Part model, mm, in its own coordinate system. A direction names the side the tool comes from. Give positions to 0.01 mm unless a question says otherwise; leave off trailing zeros. Order: outer loops, then holes, each group sorted by start corner. A loop starts at its lowest first (then second) coordinate and runs counter-clockwise, first axis right, second up. Notation, with made-up numbers: (58, 54) - (101, 54) arc R21 ccw to (101, 72) - close; hole circle Ø11 at (80.5, 18.25). An arc over 180 degrees is marked (long way). Use a Markdown table: item, result. Add a question column.
from build123d import *

# Parameters (mm, degrees)
SKETCH1_W           = 23.83
SKETCH1_H           = 1
BOSS_EXTRUDE1_DEPTH = 21.5
SKETCH2_R           = 1.325
BOSS_EXTRUDE2_DEPTH = 14.25
BOSS_EXTRUDE4_DEPTH = 8
SKETCH5_W           = 21.949336604
SKETCH5_H           = 2.5
BOSS_EXTRUDE5_DEPTH = 50
SKETCH6_R           = 4.25
SKETCH6_R_2         = 1.05
CUT_EXTRUDE1_DEPTH  = 83.099025573
FILLET1_R           = 7
FILLET2_R           = 7
FILLET3_R           = 7
BOSS_EXTRUDE6_START = 41
BOSS_EXTRUDE6_DEPTH = 41


with BuildPart() as part:
    # Sketch1 → Boss-Extrude1 (new body)
    with BuildSketch(Plane(origin=(0, 0, 0), x_dir=(1, 0, 0), z_dir=(0, 1, 0))):
        Rectangle(SKETCH1_W, SKETCH1_H)
    extrude(amount=BOSS_EXTRUDE1_DEPTH)

    # Sketch2 → Boss-Extrude2 (add, symmetric)
    with BuildSketch(Plane(origin=(0, 10.75, 0), x_dir=(1, 0, 0), z_dir=(0, 1, 0))):
        with Locations(Location((-11.915, 0, 0), (0, 0, 270))):
            Circle(SKETCH2_R)
        with Locations(Location((11.915, 0, 0), (0, 0, 270))):
            Circle(SKETCH2_R)
    extrude(amount=BOSS_EXTRUDE2_DEPTH, both=True)

    # Sketch4 → Boss-Extrude4 (add, symmetric)
    with BuildSketch(Plane(origin=(0, 0, 0), x_dir=(0, 0, -1), z_dir=(1, 0, 0))):
        Polygon((-0.5, 17.927447783), (-0.5, 21.5), (-12.5, 33.75), (-35.5, 33.75), (-35.5, 31.25), (-13.550663396, 31.25), align=None)
        Polygon((-0.5, 0), (-0.5, 3.572552217), (-13.550663396, -9.75), (-35.5, -9.75), (-35.5, -12.25), (-12.5, -12.25), align=None)
    extrude(amount=BOSS_EXTRUDE4_DEPTH, both=True)

    # Sketch5 → Boss-Extrude5 (add)
    with BuildSketch(Plane.ZY.offset(8)):
        with Locations((24.525331698, 32.5)):
            Rectangle(SKETCH5_W, SKETCH5_H)
        with Locations((24.525331698, -11)):
            Rectangle(SKETCH5_W, SKETCH5_H)
    extrude(amount=BOSS_EXTRUDE5_DEPTH)

    # Sketch6 → Cut-Extrude1 (cut, through all)
    with BuildSketch(Plane(origin=(0, 33.75, 0), x_dir=(1, 0, 0), z_dir=(0, 1, 0))):
        with Locations(Location((-47.025331698, -24.525331698, 0), (0, 0, 270))):
            Circle(SKETCH6_R)
        with Locations(Location((-54.025331698, -24.525331698, 0), (0, 0, 270))):
            Circle(SKETCH6_R_2)
        with Locations(Location((-47.025331698, -17.525331698, 0), (0, 0, 270))):
            Circle(SKETCH6_R_2)
        with Locations(Location((-40.025331698, -24.525331698, 0), (0, 0, 270))):
            Circle(SKETCH6_R_2)
        with Locations(Location((-47.025331698, -31.525331698, 0), (0, 0, 270))):
            Circle(SKETCH6_R_2)
        with BuildLine():
            ThreePointArc((-58, -24.525331743), (-54.785594092, -16.765069336), (-47.025331698, -13.550663396))
            Line((-47.025331698, -13.550663396), (-58, -13.550663396))
            Line((-58, -13.550663396), (-58, -24.525331743))
        make_face()
        with BuildLine():
            ThreePointArc((-47.025331698, -35.5), (-54.78559406, -32.285594092), (-58, -24.525331743))
            Line((-58, -24.525331743), (-58, -35.5))
            Line((-58, -35.5), (-47.025331698, -35.5))
        make_face()
    extrude(amount=-CUT_EXTRUDE1_DEPTH, mode=Mode.SUBTRACT)

    # Fillet1
    # the kernel refuses this fillet: 7 mm, written as the material it adds along each edge
    with BuildSketch(Plane(origin=(-8, -12.25, 13.550663396), x_dir=(-1, 0, 0), z_dir=(0, 1, 0))) as fillet1_piece_1_section:
        with BuildLine():
            CenterArc((FILLET1_R, -FILLET1_R), FILLET1_R, 90, 90)
            Line((0, -FILLET1_R), (0, 0))
            Line((0, 0), (FILLET1_R, 0))
        make_face()
    fillet1_piece_1 = extrude(amount=2.5, mode=Mode.PRIVATE)
    fillet1_piece_1 = split(fillet1_piece_1, bisect_by=Plane(origin=(-10.015975833, -11.661011889, 11.923032054), z_dir=(0, 0.699779834816443, 0.7143585813751185)), keep=Keep.TOP, mode=Mode.PRIVATE)
    fillet1_piece_1 = split(fillet1_piece_1, bisect_by=Plane(origin=(-10.015975833, -9.911562302, 13.708928508), z_dir=(0, -0.699779834816443, -0.7143585813751185)), keep=Keep.TOP, mode=Mode.PRIVATE)
    add(fillet1_piece_1)
    with BuildSketch(Plane(origin=(-8, -12.25, 13.550663396), x_dir=(-1, 0, 0), z_dir=(0, 1, 0))) as fillet1_piece_2_section:
        with BuildLine():
            CenterArc((FILLET1_R, -FILLET1_R), FILLET1_R, 90, 90)
            Line((0, -FILLET1_R), (0, 0))
            Line((0, 0), (FILLET1_R, 0))
        make_face()
    fillet1_piece_2 = extrude(amount=20, mode=Mode.PRIVATE)
    fillet1_piece_2 = split(fillet1_piece_2, bisect_by=Plane(origin=(-8.812454151, -9.294822672, 9.605132414), z_dir=(0, 0.699779834816443, 0.7143585813751185)), keep=Keep.TOP, mode=Mode.PRIVATE)
    fillet1_piece_2 = split(fillet1_piece_2, bisect_by=Plane(origin=(-8.812454151, -9.75, 10.768831879), z_dir=(0, 1, 0)), keep=Keep.TOP, mode=Mode.PRIVATE)
    fillet1_piece_2 = split(fillet1_piece_2, bisect_by=Plane(origin=(-8.812454151, -7.545373085, 11.391028867), z_dir=(0, -0.699779834816443, -0.7143585813751185)), keep=Keep.TOP, mode=Mode.PRIVATE)
    add(fillet1_piece_2)
    with BuildSketch(Plane(origin=(-8, 33.75, 13.550663396), x_dir=(0, 0, -1), z_dir=(0, -1, 0))) as fillet1_piece_3_section:
        with BuildLine():
            CenterArc((FILLET1_R, -FILLET1_R), FILLET1_R, 90, 90)
            Line((0, -FILLET1_R), (0, 0))
            Line((0, 0), (FILLET1_R, 0))
        make_face()
    fillet1_piece_3 = extrude(amount=2.5, mode=Mode.PRIVATE)
    fillet1_piece_3 = split(fillet1_piece_3, bisect_by=Plane(origin=(-10.015975833, 31.411562301, 13.708928507), z_dir=(0, 0.6997798348164432, -0.7143585813751182)), keep=Keep.TOP, mode=Mode.PRIVATE)
    fillet1_piece_3 = split(fillet1_piece_3, bisect_by=Plane(origin=(-10.015975833, 33.161011889, 11.923032054), z_dir=(0, -0.699779834816443, 0.7143585813751185)), keep=Keep.TOP, mode=Mode.PRIVATE)
    add(fillet1_piece_3)
    with BuildSketch(Plane(origin=(-8, 33.75, 13.550663396), x_dir=(0, 0, -1), z_dir=(0, -1, 0))) as fillet1_piece_4_section:
        with BuildLine():
            CenterArc((FILLET1_R, -FILLET1_R), FILLET1_R, 90, 90)
            Line((0, -FILLET1_R), (0, 0))
            Line((0, 0), (FILLET1_R, 0))
        make_face()
    fillet1_piece_4 = extrude(amount=20, mode=Mode.PRIVATE)
    fillet1_piece_4 = split(fillet1_piece_4, bisect_by=Plane(origin=(-8.812454159, 29.045373088, 11.39102887), z_dir=(0, 0.6997798348164432, -0.7143585813751182)), keep=Keep.TOP, mode=Mode.PRIVATE)
    fillet1_piece_4 = split(fillet1_piece_4, bisect_by=Plane(origin=(-8.812454159, 30.794822675, 9.605132416), z_dir=(0, -0.699779834816443, 0.7143585813751185)), keep=Keep.TOP, mode=Mode.PRIVATE)
    fillet1_piece_4 = split(fillet1_piece_4, bisect_by=Plane(origin=(-8.812454159, 31.25, 10.768831882), z_dir=(0, -1, 0)), keep=Keep.TOP, mode=Mode.PRIVATE)
    add(fillet1_piece_4)
    # the kernel refuses this fillet: 7 mm, written as the material it takes off along each edge
    with BuildSketch(Plane(origin=(8, 7.75, 35.5), x_dir=(0, 0, -1), z_dir=(0, -1, 0))) as fillet1_2_piece_1:
        with BuildLine():
            CenterArc((FILLET1_R, -FILLET1_R), FILLET1_R, 90, 90)
            Line((0, -FILLET1_R), (0, 0))
            Line((0, 0), (FILLET1_R, 0))
        make_face()
    extrude(amount=37.5, mode=Mode.SUBTRACT)
    with BuildSketch(Plane(origin=(8, 51.25, 35.5), x_dir=(-1, 0, 0), z_dir=(0, -1, 0))) as fillet1_2_piece_2:
        with BuildLine():
            CenterArc((FILLET1_R, FILLET1_R), FILLET1_R, 180, 90)
            Line((0, FILLET1_R), (0, 0))
            Line((0, 0), (FILLET1_R, 0))
        make_face()
    extrude(amount=37.5, mode=Mode.SUBTRACT)

    # Fillet2
    fillet2_edges = [part.edges().sort_by_distance(p)[0] for p in [
        (0, 17.927447783, 0.5),
        (0, 3.572552217, 0.5),
    ]]
    fillet(fillet2_edges, radius=FILLET2_R)

    # Fillet3
    # the kernel refuses this fillet: 7 mm, written as the material it adds along each edge
    with BuildSketch(Plane(origin=(-8, 21.5, 0.5), x_dir=(0, 0.7143585813744706, 0.6997798348171044), z_dir=(1, 0, 0))) as fillet3_piece_1:
        with BuildLine():
            CenterArc((2.380920079, -7), FILLET3_R, 90, 26.110260914)
            Line((-0.699779835, -0.714358581), (0, 0))
            Line((0, 0), (2.380920079, 0))
        make_face()
    extrude(amount=16)
    with BuildSketch(Plane(origin=(8, 0, 0.5), x_dir=(0, 0, -1), z_dir=(-1, 0, 0))) as fillet3_piece_2:
        with BuildLine():
            CenterArc((3.33439021, 6.599289533), FILLET3_R, 224.409342785, 26.110260914)
            Line((-1.666119859, 1.70083069), (0, 0))
            Line((0, 0), (1, 0))
        make_face()
    extrude(amount=16)

    # Sketch8 → Boss-Extrude6 (add)
    with BuildSketch(Plane(origin=(0, -9.75, 0), x_dir=(1, 0, 0), z_dir=(0, 1, 0)).offset(BOSS_EXTRUDE6_START)):
        with BuildLine():
            ThreePointArc((1, -35.5), (5.949747468, -33.449747468), (8, -28.5))
            Line((8, -28.5), (5, -28.5))
            ThreePointArc((5, -28.5), (3.422054899, -30.922054899), (1, -32.5))
            Line((1, -32.5), (1, -35.5))
        make_face()
    extrude(amount=-BOSS_EXTRUDE6_DEPTH)


solid = part.part
1. Pin check, flat tips, straight feed: P1, Ø10, axis at x = -11.5, z = 4.5, coming from the -Y side; P2, Ø15, axis at y = 0, z = 10, coming from the +X side; P3, Ø6.5, axis at x = -2, y = 9.5, coming from the -Z side; P4, Ø1.9, axis at x = -54.03, z = 24.53, coming from the -Y side. Stop position of each tip, or through.
2. Cut at A-A (x = -19). Write the cut outline in (y, z).
3. Cut at C-C (y = 17.5). Write the cut outline in (x, z) (3 decimals).
4. Cut at D-D (x = -5). Write the cut outline in (y, z).
5. Tool access for faces 1 (the face through (-0.11, 22.21, 0.95)), 2 (the face through (-0.112, 17.751, 1.034)), 3 (the face through (-31, 32, 13.551)), 4 (the face through (7, 11, 28.5)): list every direction of +Z, -Z, +X, -X, +Y, -Y with a clear straight run to the whole face (end or side of a thin tool).
6. Drill centre lines: probe 1 along Y at (x, z) = (3, 29); probe 2 along Y at (x, z) = (9, 0); probe 3 along Z at (x, y) = (4, 4). Where is each one in solid material? Low to high. Write a range as [from, to].
7. Mould opens along Y. For faces 5 (the face through (-23, -11, 35.5)), 6 (the face through (-12, -3.5, 0)), 7 (the face through (3.451, 11.037, 30.893)) say: released by +Y, released by -Y, zero draft, split by the parting line, or undercut.
8. Cut at B-B (z = 8). Write the cut outline in (x, y).
Responses:
| question | item | result |
|---|---|---|
| 1 | P1 | stops at y = -7.93 |
| 1 | P2 | stops at x = 8 |
| 1 | P3 | stops at z = -0.5 |
| 1 | P4 | passes through |
| 2 | outline | (-12.25, 13.55) - (-9.75, 13.55) - (-9.75, 35.5) - (-12.25, 35.5) - close; (31.25, 13.55) - (33.75, 13.55) - (33.75, 35.5) - (31.25, 35.5) - close |
| 3 | outline | (-10.688, -0.5) - (10.688, -0.5) arc R1.325 ccw (long way) to (10.688, 0.5) - (8, 0.5) - (8, 0.935) - (-8, 0.935) - (-8, 0.5) - (-10.688, 0.5) arc R1.325 ccw (long way) to start; (1, 32.5) arc R7 cw to (5, 28.5) - (8, 28.5) arc R7 ccw to (1, 35.5) - close |
| 4 | outline | (-12.25, 12.5) - (-1.7, 2.17) arc R7 cw to (0, -0.5) - (21.5, -0.5) arc R7 cw to (23.2, 2.17) - (33.75, 12.5) - (33.75, 35.5) - (31.25, 35.5) - (31.25, 13.55) - (19.97, 2.5) arc R7 cw to (15.07, 0.5) - (6.43, 0.5) arc R7 cw to (1.53, 2.5) - (-9.75, 13.55) - (-9.75, 35.5) - (-12.25, 35.5) - close |
| 5 | face 1 | -Z, +Y |
| 5 | face 2 | none |
| 5 | face 3 | -Z, -X, +Y, -Y |
| 5 | face 4 | +X, -X |
| 6 | probe 1 | y = [-12.25, -9.75], [31.25, 33.75] |
| 6 | probe 2 | y = [0, 21.5] |
| 6 | probe 3 | z = [-0.5, 0.94], [30.27, 34.82] |
| 7 | face 5 | zero draft |
| 7 | face 6 | released by -Y |
| 7 | face 7 | undercut |
| 8 | outline | (-8.15, -7.66) - (8, -7.66) - (8, -4.08) - (-8.15, -4.08) - close; (-8.15, 25.58) - (8, 25.58) - (8, 29.16) - (-8.15, 29.16) - close |
